```python
from build123d import *

# Parameters (mm, degrees)
F0_R      = 25
F1_DEPTH  = 4
F4_R      = 1.5
F4_R_2    = 1.1
F5_DEPTH  = 0.5
F5_TAPER  = 20
F6_ANGLE  = 20
F7_ANGLE  = 20
F8_ANGLE  = 20
F9_ANGLE  = 20
F10_ANGLE = 20
F13_R     = 0.75
F14_DEPTH = 4
F14_TAPER = -20
F15_R     = 2.206
F16_DEPTH = 3.8
F16_TAPER = 20
F3_R      = 1.6
F18_DEPTH = 1.8


with BuildPart() as f1:
    # F0 (on Front) → F1 (new body)
    with BuildSketch(Plane.XZ):
        Circle(F0_R)
    extrude(amount=-F1_DEPTH)



with BuildPart() as f5:
    # F4 (on face) → F5 (new body)
    with BuildSketch(Plane.XZ):
        with Locations((4.0694992911, 23.0792773443)):
            Circle(F4_R)
        with Locations((4.0694992911, 23.0792773443)):
            Circle(F4_R_2, mode=Mode.SUBTRACT)
    extrude(amount=F5_DEPTH, taper=F5_TAPER)


with BuildPart() as f6_1:
    # F6: copy of F5
    add(f5.part.rotate(Axis((0, 0, 0), (0, -1, 0)), F6_ANGLE))


with BuildPart() as f7_1:
    # F7: copy of F6_1
    add(f6_1.part.rotate(Axis((0, 0, 0), (0, -1, 0)), F7_ANGLE))


with BuildPart() as f8_1:
    # F8: copy of F7_1
    add(f7_1.part.rotate(Axis((0, 0, 0), (0, -1, 0)), F8_ANGLE))


with BuildPart() as f9_1:
    # F9: copy of F8_1
    add(f8_1.part.rotate(Axis((0, 0, 0), (0, -1, 0)), F9_ANGLE))


with BuildPart() as f10_1:
    # F10: copy of F9_1
    add(f9_1.part.rotate(Axis((0, 0, 0), (0, -1, 0)), F10_ANGLE))


with BuildPart() as f11_1:
    # F11: instance of F5
    add(f5.part.mirror(Plane.XY))


with BuildPart() as f11_2:
    # F11: instance of F6_1
    add(f6_1.part.mirror(Plane.XY))


with BuildPart() as f11_3:
    # F11: instance of F7_1
    add(f7_1.part.mirror(Plane.XY))


with BuildPart() as f11_4:
    # F11: instance of F8_1
    add(f8_1.part.mirror(Plane.XY))


with BuildPart() as f11_5:
    # F11: instance of F9_1
    add(f9_1.part.mirror(Plane.XY))


with BuildPart() as f11_6:
    # F11: instance of F10_1
    add(f10_1.part.mirror(Plane.XY))


with BuildPart() as f1_1:
    add(f1.part)

    add(f5.part)  # F12 merges F5

    add(f6_1.part)  # F12 merges F6_1

    add(f7_1.part)  # F12 merges F7_1

    add(f8_1.part)  # F12 merges F8_1

    add(f9_1.part)  # F12 merges F9_1

    add(f10_1.part)  # F12 merges F10_1

    add(f11_1.part)  # F12 merges F11_1

    add(f11_2.part)  # F12 merges F11_2

    add(f11_3.part)  # F12 merges F11_3

    add(f11_4.part)  # F12 merges F11_4

    add(f11_5.part)  # F12 merges F11_5

    add(f11_6.part)  # F12 merges F11_6
    # F12: F11_3, F11_4, F11_5, F10_1, F9_1, F8_1, F7_1 across plane
    add(f11_3.part.mirror(Plane.YZ))
    add(f11_4.part.mirror(Plane.YZ))
    add(f11_5.part.mirror(Plane.YZ))
    add(f10_1.part.mirror(Plane.YZ))
    add(f9_1.part.mirror(Plane.YZ))
    add(f8_1.part.mirror(Plane.YZ))
    add(f7_1.part.mirror(Plane.YZ))

    # F15 (on face) → F16 (cut)
    with BuildSketch(Plane(origin=(0, 4, 0), x_dir=(-1, 0, 0), z_dir=(0, 1, 0))):
        with Locations((0, -10.5)):
            Circle(F15_R)
    extrude(amount=-F16_DEPTH, taper=F16_TAPER, mode=Mode.SUBTRACT)


with BuildPart() as f14:
    # F13 (on face) → F14 (new body)
    with BuildSketch(Plane.XZ):
        with Locations((0, 10.5)):
            Circle(F13_R)
    extrude(amount=-F14_DEPTH, taper=F14_TAPER)


with BuildPart() as f1_2:
    add(f1_1.part)

    # F17: cut F14
    add(f14.part, mode=Mode.SUBTRACT)

    # F3 (on face) → F18 (cut)
    with BuildSketch(Plane.XZ):
        with Locations((6.5, 0)):
            Circle(F3_R)
        with Locations((0, 6.5)):
            Circle(F3_R)
    extrude(amount=-F18_DEPTH, mode=Mode.SUBTRACT)


solid = f1_2.part
```
Model file for the job. Use its own axes, mm. A direction names the side the tool comes from. Coordinates: 2 decimals unless noted, no trailing zeros. Write each loop counter-clockwise with the first axis right and the second up, starting at its lowest first coordinate (ties: lowest second). Pieces come first, ordered by that corner, then holes. Notation, with made-up numbers: (-2, -14) - (44, -14) arc R7 ccw to (44, -4) - close; hole circle Ø11 at (82.25, 78.5). An arc over 180 degrees is marked (long way). One line per question, with ' | ' between items. Start each with the question number.
Q1. Pull direction X, two halves, no side cores. Call faces 1 (the face through (0, 4, 0)), 2 (the face through (-22, 0, 8)): pulls with the +X half, pulls with the -X half, needs draft (parallel to the pull), parting line crosses it, or undercut.
Q2. Cut at B-B, the plane x = 0. List the corners of the cut face in (y, z).
Q3. Pin check, flat tips, straight feed: pin 1 (0.7 mm diameter, centred on x = -18.5, z = -15, fed in from -Y); pin 2 (1 mm diameter, centred on x = -16.5, y = 2.5, fed in from -Z); pin 3 (1.5 mm diameter, centred on x = 9.5, y = 1, fed in from +Z). Stop position of each tip, or through.
Q4. Drill centre lines: line 1 (Z direction, x = 0, y = 1.3); line 2 (Y direction, x = -5, z = -19); line 3 (X direction, y = 1, z = 4.5). Where is each one in solid material? Low to high. Write a range as [from, to].
Q5. Cut at C-C, the plane y = 0.8. List the corners of the cut face in (x, z).
Q6. 3-axis set-ups, long thin cutter, end or side, ignore diameter. For faces 3 (the face through (12, 0, 20)), 4 (the face through (0, 0.2, -10)): which of +Z, -Z, +X, -X, +Y, -Y reach the whole face in a straight line?
Answer below:
1) face 1: needs draft | face 2: undercut
2) outline: (0, -25) - (4, -25) - (4, -12.71) - (0.2, -11.32) - (0.2, -9.68) - (4, -8.29) - (4, 8.29) - (0, 9.75) - (0, 8.1) - (1.8, 8.1) - (1.8, 4.9) - (0, 4.9) - close; (0, 11.25) - (4, 12.71) - (4, 25) - (0, 25) - close
3) pin 1: y = 0 | pin 2: z = -19.21 | pin 3: z = 23.42
4) line 1: [-25, -11.72], [-9.28, 4.9], [8.1, 9.28], [11.72, 25] | line 2: [0, 4] | line 3: [-24.59, 24.59]
5) outline: circle Ø50 at (0, 0); hole circle Ø3.2 at (0, 6.5); hole circle Ø2.08 at (0, -10.5); hole circle Ø2.08 at (0, 10.5); hole circle Ø3.2 at (6.5, 0)
6) face 3: -Y | face 4: +Y
